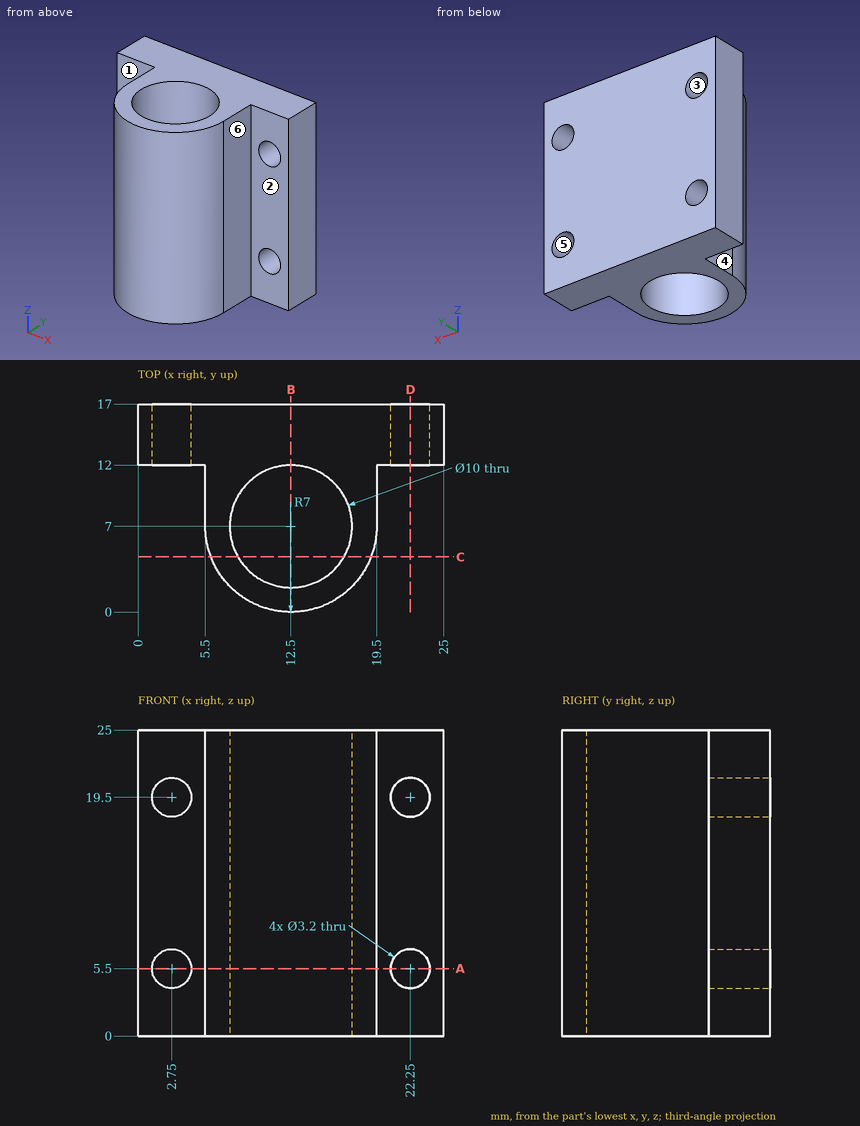
Verification items for this drawing (mm, ordinates from the low corner). A direction names the side the tool comes from. Give positions to 0.01 mm unless a question says otherwise; leave off trailing zeros. Order: outer loops, then holes, each group sorted by start corner. A loop starts at its lowest first (then second) coordinate and runs counter-clockwise, first axis right, second up.
1) Cross-section at D-D (x = 22.25). Record the boundary of the cut face in (y, z), then the cut area to 3 significant figures.
Results are:
outline: (12, 0) - (17, 0) - (17, 3.9) - (12, 3.9) - close; (12, 7.1) - (17, 7.1) - (17, 17.9) - (12, 17.9) - close; (12, 21.1) - (17, 21.1) - (17, 25) - (12, 25) - close
area: 93.0 mm2
2) Draft check along X on the marked faces 4, 5 and 6. Enter one of: released by +X, released by -X, zero draft, split by the parting line, or undercut.
Results are:
face 4: released by -X
face 5: undercut
face 6: released by +X
3) Cross-section at B-B (x = 12.5). Record the boundary of the cut face in (y, z), then the cut area to 3 significant figures.
Results are:
outline: (0, 0) - (2, 0) - (2, 25) - (0, 25) - close; (12, 0) - (17, 0) - (17, 25) - (12, 25) - close
area: 175 mm2
4) Gauge pin test, flat ends, axial feed: pin 1 (3 mm diameter, centred on x = 21.5, z = 8, fed in from -Y); pin 2 (2.5 mm diameter, centred on y = 10.5, z = 9.5, fed in from -X); pin 3 (3 mm diameter, centred on x = 2.75, z = 19.5, fed in from +Y); pin 4 (6 mm diameter, centred on y = 7.5, z = 20.5, fed in from +X). Record the tip position at first contact, or that the pin passes through.
Results are:
pin 1: stops at y = 12
pin 2: stops at x = 5.5
pin 3: passes through
pin 4: stops at x = 19.5
5) Cross-section at A-A (z = 5.5). Record the boundary of the cut face in (x, y), then the cut area to 3 significant figures.
Results are:
outline: (0, 12) - (1.15, 12) - (1.15, 17) - (0, 17) - close; (4.35, 12) - (5.5, 12) - (5.5, 7) arc R7 ccw to (19.5, 7) - (19.5, 12) - (20.65, 12) - (20.65, 17) - (4.35, 17) - close; (23.85, 12) - (25, 12) - (25, 17) - (23.85, 17) - close; hole circle Ø10 at (12.5, 7)
area: 161 mm2
6) Material ranges on probe 1 along Z at (x, y) = (2.75, 14.8); probe 2 along Y at (x, z) = (12.5, 13.5); probe 3 along X at (y, z) = (6.25, 20.75), recorded low to high.
Results are:
probe 1: z = 0 to 3.9, 7.1 to 17.9, 21.1 to 25
probe 2: y = 0 to 2, 12 to 17
probe 3: x = 5.54 to 7.56, 17.44 to 19.46
7) Cross-section at C-C (y = 4.5). Record the boundary of the cut face in (x, z).
Results are:
outline: (5.96, 0) - (8.17, 0) - (8.17, 25) - (5.96, 25) - close; (16.83, 0) - (19.04, 0) - (19.04, 25) - (16.83, 25) - close
8) Tool access check on the marked faces 1, 2 and 3. Record the directions out of +Z, -Z, +X, -X, +Y, -Y that give a thin tool (end or side, any length) a straight path to the whole face; none if there is none.
Results are:
face 1: +Z, -Z, -X, -Y
face 2: +Z, -Z, +X, -Y
face 3: +Y, -Y
